from build123d import *

# Parameters (mm, degrees)
SKETCH_1_W          = 64.5
SKETCH_1_H          = 45
EXTRUDE_1_DEPTH     = 3
SKETCH_6_W          = 12
SKETCH_6_H          = 10
EXTRUDE_4_DEPTH     = 3
FILLET_1_R          = 2
SKETCH_7_R          = 1.65
CUT_EXTRUDE_3_DEPTH = 6
SKETCH_9_W          = 6
SKETCH_9_H          = 14
CUT_EXTRUDE_4_DEPTH = 10
SKETCH_8_R          = 1.65
CUT_EXTRUDE_5_DEPTH = 10


with BuildPart() as part:
    # 草图1 → 凸台-拉伸1 (new body)
    with BuildSketch(Plane.XY):
        Rectangle(SKETCH_1_W, SKETCH_1_H)
    extrude(amount=EXTRUDE_1_DEPTH)

    # 草图6 → 凸台-拉伸4 (add)
    with BuildSketch(Plane.XY.offset(3)):
        with Locations((32.25, 0)):
            Rectangle(SKETCH_6_W, SKETCH_6_H)
        with Locations((-32.25, 0)):
            Rectangle(SKETCH_6_W, SKETCH_6_H)
    extrude(amount=-EXTRUDE_4_DEPTH)

    # 圆角1
    fillet_1_edges = [part.edges().sort_by_distance(p)[0] for p in [
        (38.25, -5, 1.5),
        (32.25, 5, 1.5),
        (32.25, -5, 1.5),
        (38.25, 5, 1.5),
        (-38.25, 5, 1.5),
        (-32.25, 5, 1.5),
        (-38.25, -5, 1.5),
        (-32.25, -5, 1.5),
        (32.25, -22.5, 1.5),
        (-32.25, -22.5, 1.5),
        (-32.25, 22.5, 1.5),
        (32.25, 22.5, 1.5),
    ]]
    fillet(fillet_1_edges, radius=FILLET_1_R)

    # 草图7 → 切除-拉伸3 (cut)
    with BuildSketch(Plane.XY.offset(3)):
        with Locations((-35.25, 0)):
            Circle(SKETCH_7_R)
        with Locations((35.25, 0)):
            Circle(SKETCH_7_R)
    extrude(amount=-CUT_EXTRUDE_3_DEPTH, mode=Mode.SUBTRACT)

    # 草图9 → 切除-拉伸4 (cut)
    with BuildSketch(Plane.XY.offset(3)):
        with Locations((-35.25, 0)):
            Rectangle(SKETCH_9_W, SKETCH_9_H)
        with Locations((35.25, 0)):
            Rectangle(SKETCH_9_W, SKETCH_9_H)
    extrude(amount=-CUT_EXTRUDE_4_DEPTH, mode=Mode.SUBTRACT)

    # 草图8 → 切除-拉伸5 (cut)
    with BuildSketch(Plane.XY.offset(3)):
        with Locations((-26.25, 0)):
            Circle(SKETCH_8_R)
        with Locations((26.25, 0)):
            Circle(SKETCH_8_R)
    extrude(amount=-CUT_EXTRUDE_5_DEPTH, mode=Mode.SUBTRACT)


solid = part.part
Build history of the part. All positions in model axes, mm. Round coordinates to 2 decimals unless told otherwise and drop trailing zeros. Loops run counter-clockwise (first coordinate to the right, second up) from the corner with the lowest first, then second, coordinate; pieces in that order, holes last. Notation, with made-up numbers: (18.25, 58.25) -> (45.25, 58.25) arc R7 cw to (45.25, 68.25) -> close; hole circle Ø6 at (26, -11). An arc over 180 degrees is marked (long way). Use CSV: the item, a comma, the result in double quotes. Start each with the question number.
Q1. Saw through at A-A on x = 26.25. Give the cut face in (y, z), and give its area (3 significant figures).
Q2. Drill centre lines: L1, parallel to X at y = 1, z = 1.2; L2, parallel to Y at x = 26.25, z = 1; L3, parallel to X at y = -1.5, z = 1.1. Where is each one in solid material? Low to high.
Q3. Mould opens along X. For faces 1 (the face through (31.65, 21.93, 1.52)), 2 (the face through (24.6, 0.07, 1.52)), 3 (the face through (0, -22.5, 1)), 4 (the face through (-27.9, 0.07, 1.52)) say: +X half, -X half, draft (parallel to the pull), parting line (faces both ways), or undercut.
Q4. Saw through at B-B on y = 0. Give the cut face in (x, z).
Solutions:
1,outline,"(-22.5, 0) -> (-1.65, 0) -> (-1.65, 3) -> (-22.5, 3) -> close; (1.65, 0) -> (22.5, 0) -> (22.5, 3) -> (1.65, 3) -> close"
1,area,"125 mm^2"
2,L1,"x = -32.25 to -27.56, -24.94 to 24.94, 27.56 to 32.25"
2,L2,"y = -22.5 to -1.65, 1.65 to 22.5"
2,L3,"x = -32.25 to -26.94, -25.56 to 25.56, 26.94 to 32.25"
3,face 1,"+X half"
3,face 2,"undercut"
3,face 3,"draft"
3,face 4,"undercut"
4,outline,"(-32.25, 0) -> (-27.9, 0) -> (-27.9, 3) -> (-32.25, 3) -> close; (-24.6, 0) -> (24.6, 0) -> (24.6, 3) -> (-24.6, 3) -> close; (27.9, 0) -> (32.25, 0) -> (32.25, 3) -> (27.9, 3) -> close"
